from build123d import *

# Parameters (mm, degrees)
F0_W           = 300
F0_H           = 300
F1_DEPTH       = 25
F4_D           = 12
F4_DEPTH       = 35.25
F4_CBORE_D     = 19.25
F4_CBORE_DEPTH = 12
F4_TIP         = 3.6051637142
F5_D           = 12
F6_D           = 20
F6_DEPTH       = 25
F6_TIP         = 6.0086061903


with BuildPart() as f1:
    # F0 (on Top) → F1 (new body)
    with BuildSketch(Plane.XY):
        Rectangle(F0_W, F0_H)
    extrude(amount=F1_DEPTH)

    # F4
    with Locations(Plane(origin=(0, 0, 0), x_dir=(1, 0, 0), z_dir=(0, 0, -1))):
        with Locations((0, -42.5), (-40.4199019425, -13.1332222609), (-24.9808732224, 34.3832222609), (24.9808732224, 34.3832222609), (40.4199019425, -13.1332222609)):
            CounterBoreHole(F4_D / 2, F4_CBORE_D / 2, F4_CBORE_DEPTH, depth=F4_DEPTH)
            with Locations((0, 0, -(F4_DEPTH + F4_TIP / 2))):  # 118° drill point
                Cone(0, F4_D / 2, F4_TIP, mode=Mode.SUBTRACT)

    # F5 (through all)
    with Locations(Plane.XY.offset(25)):
        with Locations((0, 0)):
            Hole(F5_D / 2)

    # F6
    with Locations(Plane(origin=(0, 0, 0), x_dir=(1, 0, 0), z_dir=(0, 0, -1))):
        with Locations((-120.1043392265, -106.8988462075), (-120.1043392265, -7.4011537925), (120.1043392265, -7.4011537925), (120.1043392265, -106.8988462075)):
            Hole(F6_D / 2, depth=F6_DEPTH)
            with Locations((0, 0, -(F6_DEPTH + F6_TIP / 2))):  # 118° drill point
                Cone(0, F6_D / 2, F6_TIP, mode=Mode.SUBTRACT)


solid = f1.part
Could you check a few things on this model? Use its own coordinates, in mm. A direction names the side the tool comes from. Give positions to 0.01 mm unless a question says otherwise; leave off trailing zeros. Order: outer loops, then holes, each group sorted by start corner. A loop starts at its lowest first (then second) coordinate and runs counter-clockwise, first axis right, second up.
1. Suppose I cut it at A-A (y = 42.5). List the corners of the cut face in (x, z) for me (3 decimals).
2. Will these pins go through, and if not, where does the flat tip stop? P1, Ø19, axis at x = 0, y = 42.5, coming from the -Z side; P2, Ø12, axis at x = -120.1, y = 7.4, coming from the -Z side.
3. Suppose I cut it at B-B (x = 0). List the corners of the cut face in (y, z) for me (3 decimals), plus the area to 3 significant figures.
4. Suppose I cut it at C-C (z = 8.25). Give the number of separate pieces and of enclosed holes in the cut face, plus the area to 3 significant figures.
5. We'd pull the mould along X, two halves only. Please class faces 1 (the cylindrical face through (46.414, 12.869, 18.591)), 2 (the flat face through (-150, -2, 12)), 3 (the flat face through (150, -2, 12)): pulls with the +X half, pulls with the -X half, needs draft (parallel to the pull), parting line crosses it, or undercut.
6. I need wall thicknesses on L1, parallel to Y at x = 0, z = 9 (3 decimals); L2, parallel to X at y = 15.5, z = 17.75; L3, parallel to X at y = -30, z = 12.5. Which ranges of each line are inside material? Lowest first, please.
7. For faces 4 (the flat face through (-2, 150, 12)), 5 (the cylindrical face through (-2.087, 51.896, 5.916)), which set-ups out of +Z, -Z, +X, -X, +Y, -Y let a thin tool reach every point of the face, with its end or its side?
Solved:
1. outline: (-150, 0) - (-9.625, 0) - (-9.625, 12) - (-6, 12) - (-6, 25) - (-150, 25) - close; (6, 12) - (9.625, 12) - (9.625, 0) - (150, 0) - (150, 25) - (6, 25) - close
2. P1: stops at z = 12
2. P2: passes through
3. outline: (-150, 0) - (-6, 0) - (-6, 25) - (-150, 25) - close; (6, 0) - (32.875, 0) - (32.875, 12) - (36.5, 12) - (36.5, 25) - (6, 25) - close; (48.5, 12) - (52.125, 12) - (52.125, 0) - (150, 0) - (150, 25) - (48.5, 25) - close
3. area: 6,810 mm2
4. separate pieces: 1
4. enclosed holes: 10
4. area: 87,200 mm2
5. face 1: undercut
5. face 2: pulls with the -X half
5. face 3: pulls with the +X half
6. L1: y = -150 to -6, 6 to 32.875, 52.125 to 150
6. L2: x = -150 to -125.97, -114.24 to -45.93, -34.91 to 34.91, 45.93 to 114.24, 125.97 to 150
6. L3: x = -150 to -29.08, -20.88 to 20.88, 29.08 to 150
7. face 4: +Z, -Z, +X, -X, +Y
7. face 5: -Z
